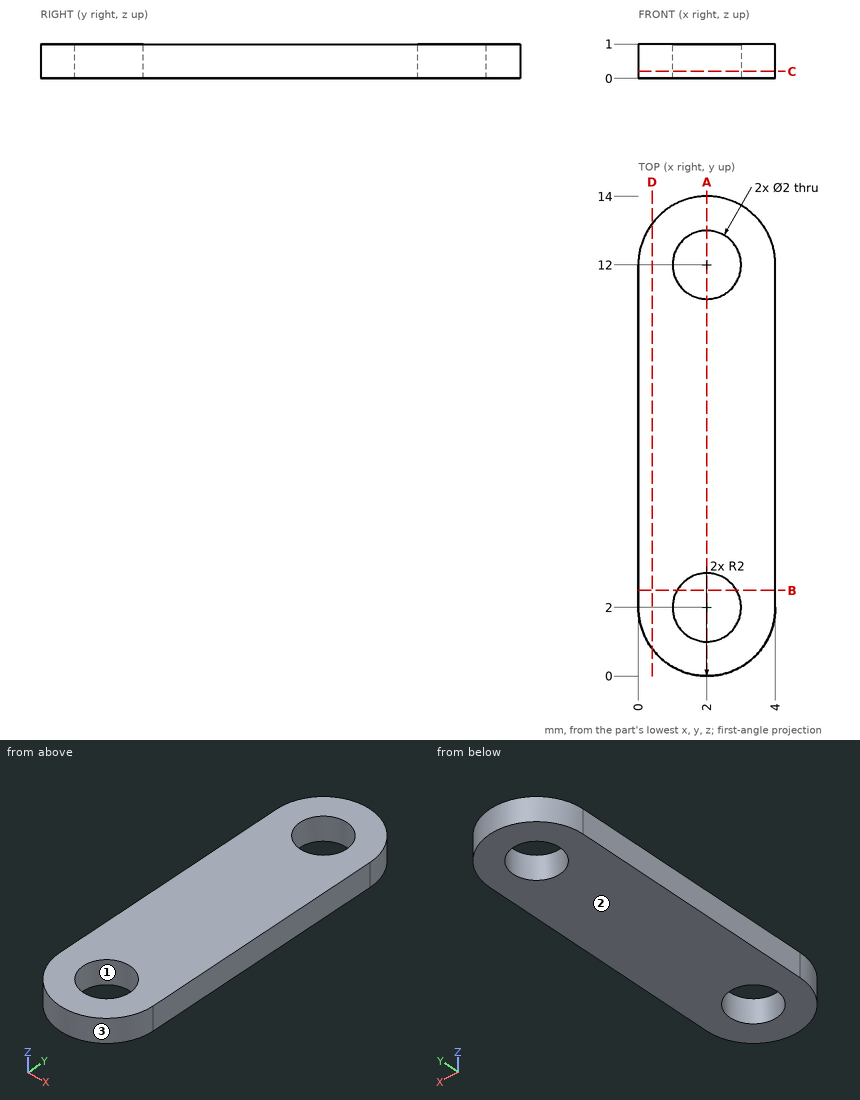
Print and shaded views of the part. All mm, measured from the part's lowest x, y and z. Give positions to 0.01 mm unless a question says otherwise; leave off trailing zeros. Write each loop counter-clockwise with the first axis right and the second up, starting at its lowest first coordinate (ties: lowest second). Pieces come first, ordered by that corner, then holes. Notation, with made-up numbers: M 27.5,0.25 L 85.5,0.25 A21 ccw 85.5,33.25 Z; hole C 4,36.25 d1. An arc over 180 degrees is marked long. Use a Markdown table: item, result.
1) Pull direction X, two halves, no side cores. Call the marked faces 1, 2 and 3: +X half, -X half, draft (parallel to the pull), parting line (faces both ways), or undercut.
Responses:
| item | result |
|---|---|
| face 1 | undercut |
| face 2 | draft |
| face 3 | parting line |
2) Cut at D-D (x = 0.4). List the corners of the cut face in (y, z).
Responses:
| item | result |
|---|---|
| outline | M 0.8,0 L 13.2,0 L 13.2,1 L 0.8,1 Z |
3) Cut at B-B (y = 2.5). List the corners of the cut face in (x, z).
Responses:
| item | result |
|---|---|
| outline | M 0,0 L 1.13,0 L 1.13,1 L 0,1 Z; M 2.87,0 L 4,0 L 4,1 L 2.87,1 Z |
4) Drill centre lines: line 1 (Y direction, x = 1.95, z = 0.8); line 2 (Y direction, x = 1.6, z = 0.85); line 3 (X direction, y = 12.25, z = 0.95). Where is each one in solid material? Low to high. Write a range as from..to.
Responses:
| item | result |
|---|---|
| line 1 | y = 0..1, 3..11, 13..14 |
| line 2 | y = 0.04..1.08, 2.92..11.08, 12.92..13.96 |
| line 3 | x = 0.02..1.03, 2.97..3.98 |
5) Cut at C-C (z = 0.2). List the corners of the cut face in (x, y), and give its area (3 significant figures).
Responses:
| item | result |
|---|---|
| outline | M 0,2 A2 ccw 4,2 L 4,12 A2 ccw 0,12 Z; hole C 2,2 d2; hole C 2,12 d2 |
| area | 46.3 mm2 |
6) Cut at A-A (x = 2). List the corners of the cut face in (y, z).
Responses:
| item | result |
|---|---|
| outline | M 0,0 L 1,0 L 1,1 L 0,1 Z; M 3,0 L 11,0 L 11,1 L 3,1 Z; M 13,0 L 14,0 L 14,1 L 13,1 Z |
